```python
from build123d import *

# Parameters (mm, degrees)
SKETCH1_W           = 76.2
SKETCH1_H           = 76.2
SKETCH1_W_2         = 69.85
SKETCH1_H_2         = 69.85
BOSS_EXTRUDE1_DEPTH = 381
SKETCH2_R           = 14.2875
SKETCH2_R_2         = 9.525
SKETCH2_R_3         = 2.4892
CUT_EXTRUDE1_DEPTH  = 304.8
SKETCH3_R           = 33.3375
CUT_EXTRUDE2_DEPTH  = 47.625
SKETCH5_R           = 14.2875
SKETCH5_R_2         = 9.525
CUT_EXTRUDE3_DEPTH  = 83.185
SKETCH6_R           = 33.3375
CUT_EXTRUDE4_DEPTH  = 47.625
SKETCH7_R           = 2.4892
CUT_EXTRUDE5_DEPTH  = 47.625
SKETCH10_R          = 3.2639
CUT_EXTRUDE7_DEPTH  = 391.408824183


with BuildPart() as part:
    # Sketch1 → Boss-Extrude1 (new body)
    with BuildSketch(Plane(origin=(0, 0, 0), x_dir=(1, 0, 0), z_dir=(0, 1, 0))):
        Rectangle(SKETCH1_W, SKETCH1_H)
        Rectangle(SKETCH1_W_2, SKETCH1_H_2, mode=Mode.SUBTRACT)
    extrude(amount=BOSS_EXTRUDE1_DEPTH)

    # Sketch2 → Cut-Extrude1 (cut)
    with BuildSketch(Plane(origin=(0, 0, -38.1), x_dir=(-1, 0, 0), z_dir=(0, 0, -1))):
        with Locations((0, 355.6)):
            Circle(SKETCH2_R)
        with Locations((0, 127)):
            Circle(SKETCH2_R_2)
        with Locations((0, 152.4)):
            Circle(SKETCH2_R_3)
        with Locations((12.7, 148.997045256)):
            Circle(SKETCH2_R_3)
        with Locations((21.997045256, 139.7)):
            Circle(SKETCH2_R_3)
        with Locations((25.4, 127)):
            Circle(SKETCH2_R_3)
        with Locations((21.997045256, 114.3)):
            Circle(SKETCH2_R_3)
        with Locations((12.7, 105.002954744)):
            Circle(SKETCH2_R_3)
        with Locations((0, 101.6)):
            Circle(SKETCH2_R_3)
        with Locations((-12.7, 105.002954744)):
            Circle(SKETCH2_R_3)
        with Locations((-21.997045256, 114.3)):
            Circle(SKETCH2_R_3)
        with Locations((-25.4, 127)):
            Circle(SKETCH2_R_3)
        with Locations((-21.997045256, 139.7)):
            Circle(SKETCH2_R_3)
        with Locations((-12.7, 148.997045256)):
            Circle(SKETCH2_R_3)
    extrude(amount=-CUT_EXTRUDE1_DEPTH, mode=Mode.SUBTRACT)

    # Sketch3 → Cut-Extrude2 (cut)
    with BuildSketch(Plane.XY.offset(38.1)):
        with Locations((0, 127)):
            Circle(SKETCH3_R)
    extrude(amount=-CUT_EXTRUDE2_DEPTH, mode=Mode.SUBTRACT)

    # Sketch5 → Cut-Extrude3 (cut)
    with BuildSketch(Plane(origin=(0, 0, -38.1), x_dir=(-1, 0, 0), z_dir=(0, 0, -1))):
        with Locations((-15.875, 294.037693501)):
            Circle(SKETCH5_R)
        with Locations((15.875, 254.284388904)):
            Circle(SKETCH5_R)
        with Locations((0, 225.244023385)):
            Circle(SKETCH5_R_2)
    extrude(amount=-CUT_EXTRUDE3_DEPTH, mode=Mode.SUBTRACT)

    # Sketch6 → Cut-Extrude4 (cut)
    with BuildSketch(Plane(origin=(0, 0, -38.1), x_dir=(-1, 0, 0), z_dir=(0, 0, -1))):
        with Locations((0, 225.244023385)):
            Circle(SKETCH6_R)
    extrude(amount=-CUT_EXTRUDE4_DEPTH, mode=Mode.SUBTRACT)

    # Sketch7 → Cut-Extrude5 (cut)
    with BuildSketch(Plane.XY.offset(38.1)):
        with Locations((0, 199.844023385)):
            Circle(SKETCH7_R)
        with Locations((-12.7, 203.246978129)):
            Circle(SKETCH7_R)
        with Locations((-21.997045256, 212.544023385)):
            Circle(SKETCH7_R)
        with Locations((-25.4, 225.244023385)):
            Circle(SKETCH7_R)
        with Locations((12.7, 247.241068641)):
            Circle(SKETCH7_R)
        with Locations((21.997045256, 237.944023385)):
            Circle(SKETCH7_R)
        with Locations((25.4, 225.244023385)):
            Circle(SKETCH7_R)
        with Locations((21.997045256, 212.544023385)):
            Circle(SKETCH7_R)
        with Locations((12.7, 203.246978129)):
            Circle(SKETCH7_R)
    extrude(amount=-CUT_EXTRUDE5_DEPTH, mode=Mode.SUBTRACT)

    # Sketch10 → Cut-Extrude7 (cut, through all)
    with BuildSketch(Plane.ZY.offset(38.1)):
        with Locations((-25.4, 12.7)):
            Circle(SKETCH10_R)
        with Locations((0, 12.7)):
            Circle(SKETCH10_R)
        with Locations((25.4, 12.7)):
            Circle(SKETCH10_R)
        with Locations((0, 38.1)):
            Circle(SKETCH10_R)
        with Locations((25.4, 38.1)):
            Circle(SKETCH10_R)
        with Locations((-25.4, 38.1)):
            Circle(SKETCH10_R)
    extrude(amount=-CUT_EXTRUDE7_DEPTH, mode=Mode.SUBTRACT)


solid = part.part
```
Verification items for the finished model (mm, model axes). A direction names the side the tool comes from. Coordinates: 2 decimals unless noted, no trailing zeros. Order: outer loops, then holes, each group sorted by start corner. A loop starts at its lowest first (then second) coordinate and runs counter-clockwise, first axis right, second up. Notation, with made-up numbers: (-10.5, 68) -> (46.5, 68) arc R21 ccw to (46.5, 101) -> close; hole circle Ø2 at (66, 89). An arc over 180 degrees is marked (long way). Put each result on its own line as item: value. Start each with the question number.
1) Release check for a two-part mould opening along X. For faces 4 (the flat face through (-34.925, 188, 0)), 5 (the cylindrical face through (-36.535, 11.45, 28.415)), 6 (the flat face through (38.1, 188, 1)) record: pulls with the +X half, pulls with the -X half, needs draft (parallel to the pull), parting line crosses it, or undercut.
2) Material ranges on L1, parallel to X at y = 139.7, z = -36.8; L2, parallel to Y at x = 0, z = -36 (1 decimal); L3, parallel to Z at x = -21.5, y = 311 (3 decimals), recorded low to high.
3) Cross-section at B-B (y = 355.6). Enter the section's corners in (x, z) (1 decimal), plus the area to 3 significant figures.
4) Go/stop test with a flat-tipped pin: pin 1 (6 mm diameter, centred on y = 12.7, z = 25.4, fed in from +X). Record where the tip stops, or that it passes through.
5) Cross-section at C-C (y = 55). Enter the section's corners in (x, z) (3 decimals), plus the area to 3 significant figures.
6) Cross-section at A-A (z = -15). Enter the section's corners in (x, y) (3 decimals), plus the area to 3 significant figures.
7) Tool access check on faces 1 (the cylindrical face through (-7.227, 94.455, 36.535)), 2 (the flat face through (0, 188, -34.925)), 3 (the cylindrical face through (-14.02, 268.45, 36.49)). Record the directions out of +Z, -Z, +X, -X, +Y, -Y that give a thin tool (end or side, any length) a straight path to the whole face; none if there is none.
Geometry check:
1. face 4: undercut
1. face 5: needs draft
1. face 6: pulls with the +X half
2. L1: x = -38.1 to -24.49, -19.51 to 19.51, 24.49 to 38.1
2. L2: y = 0 to 99.1, 104.1 to 117.5, 136.5 to 149.9, 154.9 to 191.9, 258.6 to 341.3, 369.9 to 381
2. L3: z = -38.1 to -34.925, 34.925 to 38.1
3. outline: (-38.1, -38.1) -> (-14.3, -38.1) -> (-14.3, -34.9) -> (-34.9, -34.9) -> (-34.9, 34.9) -> (-14.3, 34.9) -> (-14.3, 38.1) -> (-38.1, 38.1) -> close; (14.3, -38.1) -> (38.1, -38.1) -> (38.1, 38.1) -> (14.3, 38.1) -> (14.3, 34.9) -> (34.9, 34.9) -> (34.9, -34.9) -> (14.3, -34.9) -> close
3. area: 746 mm^2
4. pin 1: passes through
5. outline: (-38.1, -38.1) -> (38.1, -38.1) -> (38.1, 38.1) -> (-38.1, 38.1) -> close; hole (-34.925, -34.925) -> (34.925, -34.925) -> (34.925, 34.925) -> (-34.925, 34.925) -> close
5. area: 927 mm^2
6. outline: (-38.1, 0) -> (-34.925, 0) -> (-34.925, 381) -> (-38.1, 381) -> close; (34.925, 0) -> (38.1, 0) -> (38.1, 381) -> (34.925, 381) -> close
6. area: 2,420 mm^2
7. face 1: +Z
7. face 2: +Y, -Y
7. face 3: +Z, -Z
